Design review of the part built by this model. Coordinates are the model's own, in mm. A direction names the side the tool comes from. Coordinates: 2 decimals unless noted, no trailing zeros. Write each loop counter-clockwise with the first axis right and the second up, starting at its lowest first coordinate (ties: lowest second). Pieces come first, ordered by that corner, then holes. Notation, with made-up numbers: (86.5, -28.75) -> (113.5, -28.75) arc R13 ccw to (113.5, -10.75) -> close; hole circle Ø7 at (-38, 45.25). An arc over 180 degrees is marked (long way). One line per question, with ' | ' between items. Start each with the question number.
Q1. For P1, Ø0.6, axis at x = 69.5, y = -46.5, coming from the +Z side; P2, Ø6, axis at y = -70.5, z = 14, coming from the +X side, all flat-tipped, find the tip position at first contact; note any pin that passes through.
Q2. Add section C-C on z = -52.5. State the section outline as (x, y) points, and give its area (3 significant figures).
Q3. Add section B-B on x = 118. State the section outline as (y, z) points.
Q4. Add section A-A on y = -67. State the section outline as (x, z) points.
Q5. Wall thickness on probe 1 along Z at (x, y) = (13, -47.5); probe 2 along Z at (x, y) = (93.5, -46); probe 3 along X at (y, z) = (-77, 17): over which ranges is each line inside the solid? List them lowest first.
Q6. For faces 1 (the flat face through (3, -50, 40.337)), 2 (the flat face through (30, 0, -35)), list the 3-axis set-ups (+Z, -Z, +X, -X, +Y, -Y) from which the entire face can be reached by the end or side of a thin tool; tool diameter is ignored.
from build123d import *

# Parameters (mm, degrees)
F0_W     = 127
F0_H     = 152.4
F1_DEPTH = 101.6
F2_W     = 101.6
F2_H     = 50.8
F3_DEPTH = 101.6
F5_DEPTH = 101.6


with BuildPart() as f1:
    # F0 (on Front) → F1 (new body)
    with BuildSketch(Plane.XZ):
        with Locations((6.165242, -35.863342)):
            Rectangle(F0_W, F0_H)
    extrude(amount=F1_DEPTH)

    # F2 (on face) → F3 (join)
    with BuildSketch(Plane.YZ.offset(69.665242)):
        with Locations((-50.8, -86.663342)):
            Rectangle(F2_W, F2_H)
    extrude(amount=F3_DEPTH)

    # F4 (on Front) → F5 (join)
    with BuildSketch(Plane.XZ):
        Polygon((68.383813, 40.888175), (-30.263531, 17.656446), (67.372276, -89.133667), (170.625895, -61.112218), align=None)
    extrude(amount=F5_DEPTH)


solid = f1.part
Output values:
1) P1: stops at z = 40.34 | P2: stops at x = 98.34
2) outline: (-57.33, -101.6) -> (161.99, -101.6) -> (161.99, 0) -> (-57.33, 0) -> close | area: 22,300 mm2
3) outline: (-101.6, -112.06) -> (0, -112.06) -> (0, -8.61) -> (-101.6, -8.61) -> close
4) outline: (-57.33, -112.06) -> (171.27, -112.06) -> (171.27, -61.26) -> (170.07, -61.26) -> (170.63, -61.11) -> (69.67, 39.61) -> (69.67, 40.34) -> (68.94, 40.34) -> (68.38, 40.89) -> (66.04, 40.34) -> (-57.33, 40.34) -> close
5) probe 1: z = -112.06 to 40.34 | probe 2: z = -112.06 to 15.83 | probe 3: x = -57.33 to 92.33
6) face 1: +Z, -X, +Y, -Y | face 2: +Z, -Z, +X, -X, +Y
